Could you check a few things on this drawing? It's one solid part, dimensions in mm from its lowest x, y, z. Give positions to 0.01 mm unless a question says otherwise; leave off trailing zeros. Order: outer loops, then holes, each group sorted by start corner. A loop starts at its lowest first (then second) coordinate and runs counter-clockwise, first axis right, second up. Notation, with made-up numbers: (24.25, 12) - (70.25, 12) arc R24 cw to (70.25, 34) - close; hole circle Ø9 at (5.5, -32). An arc over 180 degrees is marked (long way). Answer as CSV lines item,"result".
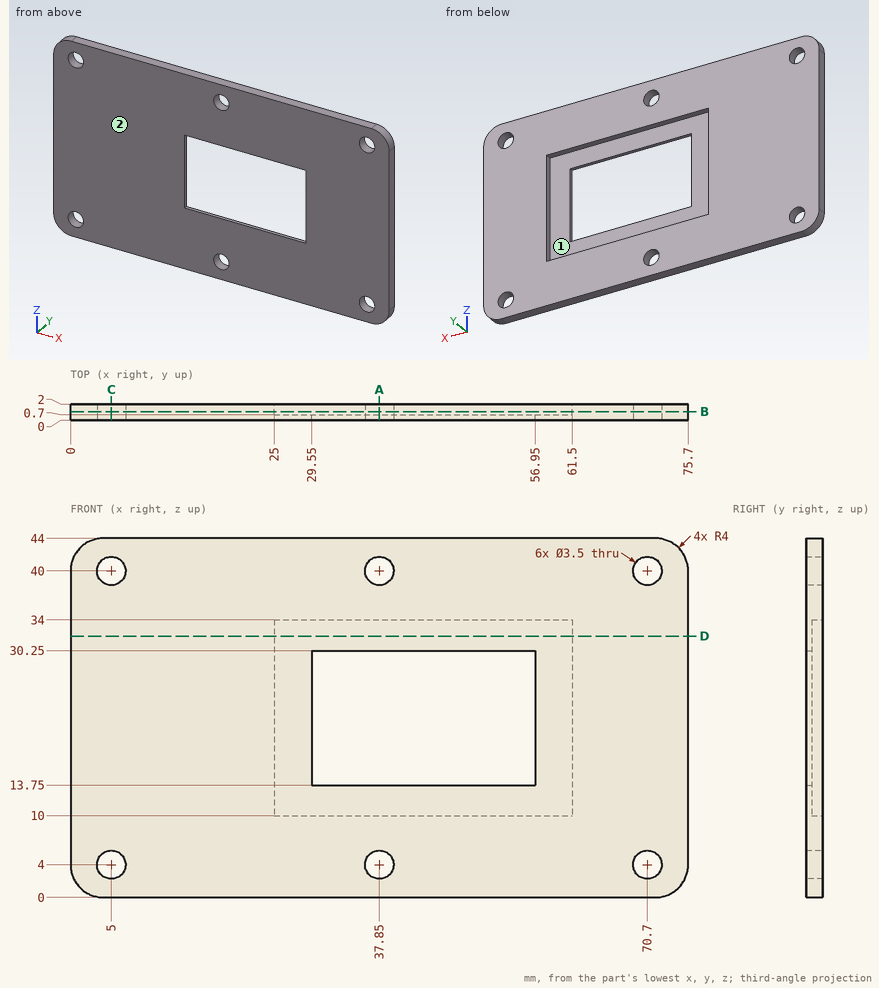
1) I want a section at D-D on z = 32. Write out the boundary of the cut face in (x, y), plus the area to 3 significant figures.
Answer block:
outline,"(0, 0) - (75.7, 0) - (75.7, 2) - (61.5, 2) - (61.5, 0.7) - (25, 0.7) - (25, 2) - (0, 2) - close"
area,"104 mm2"
2) I want a section at C-C on x = 5. Write out the boundary of the cut face in (y, z).
Answer block:
outline,"(0, 0) - (2, 0) - (2, 2.25) - (0, 2.25) - close; (0, 5.75) - (2, 5.75) - (2, 38.25) - (0, 38.25) - close; (0, 41.75) - (2, 41.75) - (2, 44) - (0, 44) - close"
3) I want a section at A-A on x = 37.85. Write out the boundary of the cut face in (y, z), plus the area to 4 significant figures.
Answer block:
outline,"(0, 0) - (2, 0) - (2, 2.25) - (0, 2.25) - close; (0, 5.75) - (2, 5.75) - (2, 10) - (0.7, 10) - (0.7, 13.75) - (0, 13.75) - close; (0, 30.25) - (0.7, 30.25) - (0.7, 34) - (2, 34) - (2, 38.25) - (0, 38.25) - close; (0, 41.75) - (2, 41.75) - (2, 44) - (0, 44) - close"
area,"31.25 mm2"
4) If we mould it in two halves opening along Z, with no side actions, what happens to the marked faces 1 and 2? For each: +Z half, -Z half, draft (parallel to the pull), parting line (faces both ways), or undercut.
Answer block:
face 1,"undercut"
face 2,"draft"
5) I'm going to push a flat-ended pin straight in: P1, Ø1, axis at x = 45.5, z = 31.5, coming from the +Y side. Where does the tip first touch, or does it pass through?
Answer block:
P1,"y = 0.7"
6) I want a section at B-B on y = 1.05. Write out the boundary of the cut face in (x, z), plus the area to 3 significant figures.
Answer block:
outline,"(0, 4) arc R4 ccw to (4, 0) - (71.7, 0) arc R4 ccw to (75.7, 4) - (75.7, 40) arc R4 ccw to (71.7, 44) - (4, 44) arc R4 ccw to (0, 40) - close; hole circle Ø3.5 at (5, 4); hole circle Ø3.5 at (5, 40); hole (25, 10) - (61.5, 10) - (61.5, 34) - (25, 34) - close; hole circle Ø3.5 at (37.85, 4); hole circle Ø3.5 at (37.85, 40); hole circle Ø3.5 at (70.7, 4); hole circle Ø3.5 at (70.7, 40)"
area,"2,380 mm2"
7) I need wall thicknesses on line 1 along X through (y, z) = (0.85, 4); line 2 along Z through (x, y) = (70.7, 0.5); line 3 along Z through (x, y) = (38.5, 0.1). Which ranges of each line are inside material? Lowest first, please. Write a range as [from, to].
Answer block:
line 1,"[0, 3.25], [6.75, 36.1], [39.6, 68.95], [72.45, 75.7]"
line 2,"[0, 2.25], [5.75, 38.25], [41.75, 44]"
line 3,"[0, 2.38], [5.62, 13.75], [30.25, 38.38], [41.62, 44]"
